```python
from build123d import *

# Parameters (mm, degrees)
SKETCH_R     = 2.75
PAD_DEPTH    = 2
SKETCH001_R  = 1.45
PAD001_DEPTH = 4
FILLET_R     = 1


with BuildPart() as part:
    # Sketch → Pad (new body)
    with BuildSketch(Plane.XY):
        Circle(SKETCH_R)
    extrude(amount=PAD_DEPTH)

    # Sketch001 (on Face3 of Pad) → Pad001 (join)
    with BuildSketch(Plane.XY.offset(2)):
        Circle(SKETCH001_R)
    extrude(amount=PAD001_DEPTH)

    # Fillet
    fillet_edges = [part.edges().sort_by_distance(p)[0] for p in [
        (-1.45, 0, 6),
    ]]
    fillet(fillet_edges, radius=FILLET_R)


solid = part.part
```
Part model, mm, in its own coordinate system. A direction names the side the tool comes from. Coordinates: 2 decimals unless noted, no trailing zeros. Write each loop counter-clockwise with the first axis right and the second up, starting at its lowest first coordinate (ties: lowest second). Pieces come first, ordered by that corner, then holes.
Item 1: Slice it at A-A (z = 0.5). Write the cut outline in (x, y), and give its area (3 significant figures).
Item 2: Slice it at D-D (z = 4.45). Write the cut outline in (x, y).
Item 3: Which spindle directions (+Z, -Z, +X, -X, +Y, -Y) get a long thin tool onto all of the face, cutting with end or side? Do faces 1 (the face through (0, 0, 6)), 2 (the face through (1.2, -1.2, 2)). Say none if no direction does.
Item 4: Slice it at C-C (x = 1.55). Write the cut outline in (y, z).
Item 5: Slice it at B-B (y = -1.7). Write the cut outline in (x, z), and give its area (3 significant figures).
Item 6: Probe line 1 (Z direction, x = 1.35, y = -2); line 2 (X direction, y = -0.05, z = 5.05); line 3 (X direction, y = -0.15, z = 0.65). List the from-to ranges inside material, lowest first.
Item 7: Pin check, flat tip, straight feed: pin 1 (1 mm diameter, centred on y = -1, z = 1.5, fed in from +X). Stop position of the tip, or through.
Results found:
1. outline: circle Ø5.5 at (0, 0)
1. area: 23.8 mm2
2. outline: circle Ø2.9 at (0, 0)
3. face 1: +Z, +X, -X, +Y, -Y
3. face 2: +Z
4. outline: (-2.27, 0) - (2.27, 0) - (2.27, 2) - (-2.27, 2) - close
5. outline: (-2.16, 0) - (2.16, 0) - (2.16, 2) - (-2.16, 2) - close
5. area: 8.65 mm2
6. line 1: z = 0 to 2
6. line 2: x = -1.45 to 1.45
6. line 3: x = -2.75 to 2.75
7. pin 1: stops at x = 2.7
